from build123d import *

# Parameters (mm, degrees)
CROQUIS1_W              = 280
CROQUIS1_H              = 110
SALIENTE_EXTRUIR1_DEPTH = 6.35
CROQUIS2_R              = 3
CROQUIS2_R_2            = 15
CORTAR_EXTRUIR2_DEPTH   = 20
CROQUIS5_R              = 2
CORTAR_EXTRUIR5_DEPTH   = 30
CROQUIS6_R              = 2
CORTAR_EXTRUIR6_DEPTH   = 30


with BuildPart() as part:
    # Croquis1 → Saliente-Extruir1 (new body)
    with BuildSketch(Plane(origin=(0, 0, 0), x_dir=(1, 0, 0), z_dir=(0, 1, 0))):
        with Locations((14.294294294, 1.756756757)):
            Rectangle(CROQUIS1_W, CROQUIS1_H)
    extrude(amount=SALIENTE_EXTRUIR1_DEPTH)

    # Croquis2 → Cortar-Extruir2 (cut)
    with BuildSketch(Plane(origin=(0, 0, 0), x_dir=(1, 0, 0), z_dir=(0, 1, 0))):
        with Locations((-39.455705706, 5.006756757)):
            Circle(CROQUIS2_R)
        with Locations((-75.955705706, 5.006756757)):
            Circle(CROQUIS2_R)
        with Locations((86.294294294, -13.243243243)):
            Circle(CROQUIS2_R_2)
        with Locations((-57.705705706, -13.243243243)):
            Circle(CROQUIS2_R_2)
        with Locations((-39.455705706, -31.493243243)):
            Circle(CROQUIS2_R)
        with Locations((-75.955705706, -31.493243243)):
            Circle(CROQUIS2_R)
        with Locations((104.544294294, 5.006756757)):
            Circle(CROQUIS2_R)
        with Locations((68.044294294, 5.006756757)):
            Circle(CROQUIS2_R)
        with Locations((104.544294294, -31.493243243)):
            Circle(CROQUIS2_R)
        with Locations((68.044294294, -31.493243243)):
            Circle(CROQUIS2_R)
    extrude(amount=CORTAR_EXTRUIR2_DEPTH, mode=Mode.SUBTRACT)

    # Croquis5 → Cortar-Extruir5 (cut)
    with BuildSketch(Plane.ZY.offset(125.705705706)):
        with Locations((38.243243243, 3.175)):
            Circle(CROQUIS5_R)
        with Locations((-41.756756757, 3.175)):
            Circle(CROQUIS5_R)
        with Locations((-1.756756757, 3.175)):
            Circle(CROQUIS5_R)
    extrude(amount=-CORTAR_EXTRUIR5_DEPTH, mode=Mode.SUBTRACT)

    # Croquis6 → Cortar-Extruir6 (cut)
    with BuildSketch(Plane(origin=(154.294294294, 0, 0), x_dir=(0, 0, -1), z_dir=(1, 0, 0))):
        with Locations((41.756756757, 3.175)):
            Circle(CROQUIS6_R)
        with Locations((-38.243243243, 3.175)):
            Circle(CROQUIS6_R)
        with Locations((1.756756757, 3.175)):
            Circle(CROQUIS6_R)
    extrude(amount=-CORTAR_EXTRUIR6_DEPTH, mode=Mode.SUBTRACT)


solid = part.part
The listing builds one solid part. Answer for the finished solid, in the listing's coordinates (mm). Give positions to 0.01 mm unless a question says otherwise; leave off trailing zeros. Write each loop counter-clockwise with the first axis right and the second up, starting at its lowest first coordinate (ties: lowest second). Pieces come first, ordered by that corner, then holes.
1) Section D-D (x = -69) is taken. Write down the section's boundary in (y, z), and give its area (3 significant figures).
2) Section A-A (x = 79.5) is taken. Write down the section's boundary in (y, z).
3) Section B-B (z = 5) is taken. Write down the section's boundary in (x, y), and give its area (3 significant figures).
4) Find the intervals of material crossed by L1, parallel to Z at x = 68.5, y = 4.25; L2, parallel to X at y = 4.5, z = -4.5; L3, parallel to X at y = 5.75, z = 23, in increasing order.
5) Given P1, Ø3, axis at y = 3.18, z = -41.76, coming from the -X side; P2, Ø3, axis at y = 3.18, z = -1.76, coming from the +X side, each flat-ended and moving along its own axis, determine where each tip first touches the part or whether it passes through.
6) For a pull along X with two mould halves and no side action, classify faces 1 (the face through (154.294, 5.2, -1)), 2 (the face through (101.547, 3.131, -5.139)), 3 (the face through (12, 0, -3)) as pulls with the +X half, pulls with the -X half, needs draft (parallel to the pull), parting line crosses it, or undercut.
7) Section C-C (x = -101) is taken. Write down the section's boundary in (y, z) (3 decimals), and give its area (3 significant figures).
Response:
1. outline: (0, -56.76) - (6.35, -56.76) - (6.35, 3.37) - (0, 3.37) - close; (0, 23.11) - (6.35, 23.11) - (6.35, 53.24) - (0, 53.24) - close
1. area: 573 mm2
2. outline: (0, -56.76) - (6.35, -56.76) - (6.35, -0.13) - (0, -0.13) - close; (0, 26.62) - (6.35, 26.62) - (6.35, 53.24) - (0, 53.24) - close
3. outline: (-125.71, 0) - (-70.24, 0) - (-70.24, 6.35) - (-125.71, 6.35) - close; (-45.17, 0) - (73.76, 0) - (73.76, 6.35) - (-45.17, 6.35) - close; (98.83, 0) - (154.29, 0) - (154.29, 6.35) - (98.83, 6.35) - close
3. area: 1,460 mm2
4. L1: z = -56.76 to -7.97, -2.04 to 28.53, 34.46 to 53.24
4. L2: x = -125.71 to -78.91, -73 to -42.41, -36.5 to 65.09, 71 to 101.59, 107.5 to 154.29
4. L3: x = -125.71 to -69.1, -46.31 to 74.9, 97.69 to 154.29
5. P1: stops at x = -95.71
5. P2: stops at x = 124.29
6. face 1: pulls with the +X half
6. face 2: undercut
6. face 3: needs draft
7. outline: (0, -56.757) - (6.35, -56.757) - (6.35, 53.243) - (0, 53.243) - close; hole circle Ø4 at (3.175, -41.757); hole circle Ø4 at (3.175, -1.757); hole circle Ø4 at (3.175, 38.243)
7. area: 661 mm2
